Verification items for the finished model (mm, model axes). A direction names the side the tool comes from. Coordinates: 2 decimals unless noted, no trailing zeros. Write each loop counter-clockwise with the first axis right and the second up, starting at its lowest first coordinate (ties: lowest second). Pieces come first, ordered by that corner, then holes. Notation, with made-up numbers: (-5.5, -14) - (27.5, -14) arc R6 ccw to (27.5, -10) - close; hole circle Ø8 at (66.25, 81). An arc over 180 degrees is marked (long way). Answer as CSV lines item,"result". Start each with the question number.
Autodesk Inventor part; units mm, degrees
ref_plane "Work Plane1" through (1.525, 0, 0) normal (0, 0, 1) x (1, 0, 0)
ref_plane "YZ Plane" through (0, 0, 0) normal (1, 0, 0) x (0, 1, 0)
ref_plane "XZ Plane" through (0, 0, 0) normal (0, 1, 0) x (-1, 0, 0)
sketch "Szkic1" plane through (0, 0, 0) normal (0, 0, 1) x (1, 0, 0)
  line L0 (0, 3.6) -> (0, 2.5)
  line L1 (6, 2.5) -> (22, 2.5)
  line L2 (22, 2.5) -> (22, 0)
  line L3 (22, 0) -> (-0.2001, 0)
  line L4 (-4.6401, 0) -> (26.44, 0)
  line L5 (-0.2001, 0) -> (-0.2001, 3.6)
  line L6 (-0.2001, 3.6) -> (0, 3.6)
  line L7 (6, 2.5) -> (5.5091, 2.5)
  line L8 (5.5091, 2.5) -> (0, 2.5)
  line L9 (0, -0.72) -> (0, 4.32)
  dimension "d0" = 22
  dimension "d1" = 16
  dimension "d2" = 5
  dimension "d9" = 0.2001
  dimension "d10" = 7.2
  dimension "d13" = 0.4909
  dimension "d14" = 5
revolve "Bryła" add sketch "Szkic1" angle 360 about axis through (22, 0, 0) along (-1, 0, 0)
sketch "Szkic2" plane through (-0.2001, 0, 0) normal (-1, 0, 0) x (0, 0, 1)
  line L0 (0, 4.6188) -> (4, 2.3094)
  line L1 (4, 2.3094) -> (4, -2.3094)
  line L2 (4, -2.3094) -> (0, -4.6188)
  line L3 (0, -4.6188) -> (-4, -2.3094)
  line L4 (-4, -2.3094) -> (-4, 2.3094)
  line L5 (-4, 2.3094) -> (0, 4.6188)
  point P0 (0, 0)
  point P1 (0, 0)
  dimension "d11" = 8
extrude "Głowica" add sketch "Szkic2" along normal blind 3.45
sketch "Szkic4" plane through (0, 0, 0) normal (0, 0, 1) x (1, 0, 0)
  line L0 (-3.6501, 4) -> (-3.6501, 4.6188)
  line L1 (-3.6501, 4.6188) -> (-3.2928, 4.6188)
  line L2 (-3.2928, 4.6188) -> (-3.6501, 4)
  line L3 (-4.3401, 0) -> (0.4899, 0)
  line L4 (-0.2001, 4.6188) -> (-3.6501, 4.6188)
  line L5 (-3.6501, 2.3094) -> (-3.6501, 4.6188)
  dimension "d5" = 30
  dimension "d19" = 8
revolve "Faza1" cut sketch "Szkic4" angle 360 about axis through (-10, 0, 0) along (1, 0, 0)
thread "Gwint"
chamfer "Faza2" distance 0.4908 distance2 0.4909 1 edges at (22, -2.5, 0) measured on face at (22, -0.7192, -0.1653)
ref_plane "Work Plane1" through (1.525, 0, 0) normal (0, 0, 1) x (1, 0, 0)
equation "\"d0\" = NLG"
equation "\"d1\" = GEL"
equation "\"d2\" = GD"
equation "\"d10\" = SD2"
equation "\"d14\" = BDM"
equation "\"d11\" = SW"
equation "\"d3\" = KOH - SD"
equation "\"d5\" = ANG1"
equation "\"d19\" = SW0"
equation "\"d15\" = GEL"
equation "\"d6\" = -0.5 * SPD + 0.5 * GD"
equation "\"NLG\" = 22"
equation "\"GD\" = NND"
equation "\"BDM\" = NND"
equation "\"KOH\" = 3.65"
equation "\"GEL\" = 16"
equation "\"SW\" = 8"
equation "\"SW0\" = 8"
equation "\"SPD\" = NND - 1.2269 * PTC"
equation "\"SD2\" = 0.9 * SW"
equation "\"SD\" = 0.2"
equation "\"ANG1\" = 30deg"
equation "\"GAL\" = 0.61345 * PTC"
equation "\"GUL\" = 0.61345 * PTC"
equation "\"RR\" = 0.35"
equation "\"GD1\" = THREADDIA - 1.2269 * PTC"
equation "\"THREADDIA\" = 5"
equation "\"SDH\" = 7.55"
equation "\"TOA\" = 30deg"
equation "\"PTC\" = 0.8"
equation "\"NND\" = 5"
equation "\"E0\" = 1.155 * SW"
properties part number "BS 3692 - M5 x 22" material "Stal, miękka"
1. Draft check along X on faces 1 (the face through (-2, 0, 4)), 2 (the face through (0, -0.9, -2.5)), 3 (the face through (-3.563, 2.084, 3.589)). Enter one of: pulls with the +X half, pulls with the -X half, needs draft (parallel to the pull), parting line crosses it, or undercut.
2. Scan lines: line 1 along Z through (x, y) = (2.25, -1.5); line 2 along X through (y, z) = (2.75, -0.75). Record each from-to range of solid material in increasing order. Write a range as from..to.
3. Cross-section at A-A (x = 11.25). Record the cut outline in (y, z), and give its area (3 significant figures).
4. Depth check by flat-ended pin: P1, Ø3, axis at x = 6, z = 1, coming from the +Y side; P2, Ø1.5, axis at x = 17, y = 2, coming from the +Z side; P3, Ø2, axis at x = 19, z = -2, coming from the -Y side. Enter the tip coordinate at first touch or a pass-through.
5. Access from +Z, -Z, +X, -X, +Y, -Y to the whole of each face (thin tool, end or side, straight path). Record for faces 4 (the face through (-0.2, -4, 0)), 5 (the face through (-3.65, 0, 0)).
Completed:
1,face 1,"needs draft"
1,face 2,"pulls with the +X half"
1,face 3,"pulls with the -X half"
2,line 1,"z = -2..2"
2,line 2,"x = -3.65..0"
3,outline,"circle Ø5 at (0, 0)"
3,area,"19.6 mm2"
4,P1,"stops at y = 2.5"
4,P2,"stops at z = 2.17"
4,P3,"stops at y = -2.29"
5,face 4,"+X"
5,face 5,"+Z, -Z, -X, +Y, -Y"
